```python
from build123d import *

# Parameters (mm, degrees)
BOSS_EXTRUDE1_START                 = 5
BOSS_EXTRUDE1_DEPTH                 = 5
BOSS_EXTRUDE2_START                 = 5
BOSS_EXTRUDE2_DEPTH                 = 5
BOSS_EXTRUDE3_START                 = 5
BOSS_EXTRUDE3_DEPTH                 = 5
F_1_5MM_DOWEL_HOLE1_D               = 1.5
F_1_5MM_DOWEL_HOLE1_DEPTH           = 3
F_1_5MM_DOWEL_HOLE1_TIP             = 0.450645464
F_1_5MM_DOWEL_HOLE1_ON_FACE_2_D     = 1.5
F_1_5MM_DOWEL_HOLE1_ON_FACE_2_DEPTH = 3
F_1_5MM_DOWEL_HOLE1_ON_FACE_2_TIP   = 0.450645464
F_1_5MM_DOWEL_HOLE1_ON_FACE_3_D     = 1.5
F_1_5MM_DOWEL_HOLE1_ON_FACE_3_DEPTH = 3
F_1_5MM_DOWEL_HOLE1_ON_FACE_3_TIP   = 0.450645464
F_1_5MM_DOWEL_HOLE1_ON_FACE_4_D     = 1.5
F_1_5MM_DOWEL_HOLE1_ON_FACE_4_DEPTH = 3
F_1_5MM_DOWEL_HOLE1_ON_FACE_4_TIP   = 0.450645464
F_1_5MM_DOWEL_HOLE1_ON_FACE_5_D     = 1.5
F_1_5MM_DOWEL_HOLE1_ON_FACE_5_DEPTH = 3
F_1_5MM_DOWEL_HOLE1_ON_FACE_5_TIP   = 0.450645464
F_1_5MM_DOWEL_HOLE1_ON_FACE_6_D     = 1.5
F_1_5MM_DOWEL_HOLE1_ON_FACE_6_DEPTH = 3
F_1_5MM_DOWEL_HOLE1_ON_FACE_6_TIP   = 0.450645464
CUT_EXTRUDE2_DEPTH                  = 4


with BuildPart() as part:
    # Sketch1 → Revolve1 (revolve)
    with BuildSketch(Plane.XY, mode=Mode.PRIVATE) as revolve1_sk:
        Polygon((54, 11), (55.5, 11), (55.5, -4), (48, -4), (48, -3), (54, -3), align=None)
    revolve(revolve1_sk.sketch.rotate(Axis((0, 0, 0), (0, 1, 0)), 90), axis=Axis((0, 0, 0), (0, 1, 0)))

    # Sketch3 → Boss-Extrude1 (add)
    with BuildSketch(Plane(origin=(0, -3, 0), x_dir=(1, 0, 0), z_dir=(0, 1, 0)).offset(BOSS_EXTRUDE1_START)):
        with BuildLine():
            Line((-16.686917696, -51.35705188), (-15.450849719, -47.552825815))
            ThreePointArc((-15.450849719, -47.552825815), (-25, -43.301270189), (-33.456530318, -37.157241274))
            Line((-33.456530318, -37.157241274), (-36.133052743, -40.129820576))
            ThreePointArc((-36.133052743, -40.129820576), (-27, -46.765371804), (-16.686917696, -51.35705188))
        make_face()
    extrude(amount=-BOSS_EXTRUDE1_DEPTH)

    # Sketch3_3 → Boss-Extrude2 (add)
    with BuildSketch(Plane(origin=(0, -3, 0), x_dir=(1, 0, 0), z_dir=(0, 1, 0)).offset(BOSS_EXTRUDE2_START)):
        with BuildLine():
            ThreePointArc((48.907380037, 10.395584541), (49.726094768, 5.226423163), (50, 0))
            ThreePointArc((50, 0), (49.726094768, -5.226423163), (48.907380037, -10.395584541))
            Line((48.907380037, -10.395584541), (52.81997044, -11.227231304))
            ThreePointArc((52.81997044, -11.227231304), (53.70418235, -5.644537016), (54, 0))
            ThreePointArc((54, 0), (53.70418235, 5.644537016), (52.81997044, 11.227231304))
            Line((52.81997044, 11.227231304), (48.907380037, 10.395584541))
        make_face()
    extrude(amount=-BOSS_EXTRUDE2_DEPTH)

    # Sketch3_4 → Boss-Extrude3 (add)
    with BuildSketch(Plane(origin=(0, -3, 0), x_dir=(1, 0, 0), z_dir=(0, 1, 0)).offset(BOSS_EXTRUDE3_START)):
        with BuildLine():
            Line((-36.133052743, 40.129820576), (-33.456530318, 37.157241274))
            ThreePointArc((-33.456530318, 37.157241274), (-25, 43.301270189), (-15.450849719, 47.552825815))
            Line((-15.450849719, 47.552825815), (-16.686917696, 51.35705188))
            ThreePointArc((-16.686917696, 51.35705188), (-27, 46.765371804), (-36.133052743, 40.129820576))
        make_face()
    extrude(amount=-BOSS_EXTRUDE3_DEPTH)

    # 1.5mm Dowel Hole1
    with Locations(Plane(origin=(-30.090751158, 0, -39.931775502), x_dir=(0.798635510047, 0, -0.601815023152), z_dir=(0.601815023152, 0, 0.798635510047))):
        with Locations((1e-09, 0)):
            Hole(F_1_5MM_DOWEL_HOLE1_D / 2, depth=F_1_5MM_DOWEL_HOLE1_DEPTH)
            with Locations((0, 0, -(F_1_5MM_DOWEL_HOLE1_DEPTH + F_1_5MM_DOWEL_HOLE1_TIP / 2))):  # 118° drill point
                Cone(0, F_1_5MM_DOWEL_HOLE1_D / 2, F_1_5MM_DOWEL_HOLE1_TIP, mode=Mode.SUBTRACT)

    # 1.5mm Dowel Hole1 on face 2
    with Locations(Plane(origin=(-19.536556424, 0, -46.025242673), x_dir=(0.92050492204, 0, -0.390730966908), z_dir=(0.390730966908, 0, 0.92050492204))):
        with Locations((-1e-09, 0)):
            Hole(F_1_5MM_DOWEL_HOLE1_ON_FACE_2_D / 2, depth=F_1_5MM_DOWEL_HOLE1_ON_FACE_2_DEPTH)
            with Locations((0, 0, -(F_1_5MM_DOWEL_HOLE1_ON_FACE_2_DEPTH + F_1_5MM_DOWEL_HOLE1_ON_FACE_2_TIP / 2))):  # 118° drill point
                Cone(0, F_1_5MM_DOWEL_HOLE1_ON_FACE_2_D / 2, F_1_5MM_DOWEL_HOLE1_ON_FACE_2_TIP, mode=Mode.SUBTRACT)

    # 1.5mm Dowel Hole1 on face 3
    with Locations(Plane(origin=(49.627307582, 0, -6.09346717), x_dir=(-0.121869023443, 0, -0.992546190928), z_dir=(-0.992546190928, 0, 0.121869023443))):
        with Locations((0, 0)):
            Hole(F_1_5MM_DOWEL_HOLE1_ON_FACE_3_D / 2, depth=F_1_5MM_DOWEL_HOLE1_ON_FACE_3_DEPTH)
            with Locations((0, 0, -(F_1_5MM_DOWEL_HOLE1_ON_FACE_3_DEPTH + F_1_5MM_DOWEL_HOLE1_ON_FACE_3_TIP / 2))):  # 118° drill point
                Cone(0, F_1_5MM_DOWEL_HOLE1_ON_FACE_3_D / 2, F_1_5MM_DOWEL_HOLE1_ON_FACE_3_TIP, mode=Mode.SUBTRACT)

    # 1.5mm Dowel Hole1 on face 4
    with Locations(Plane(origin=(49.627307582, 0, 6.09346717), x_dir=(0.121869023443, 0, -0.992546190928), z_dir=(-0.992546190928, 0, -0.121869023443))):
        with Locations((0, 0)):
            Hole(F_1_5MM_DOWEL_HOLE1_ON_FACE_4_D / 2, depth=F_1_5MM_DOWEL_HOLE1_ON_FACE_4_DEPTH)
            with Locations((0, 0, -(F_1_5MM_DOWEL_HOLE1_ON_FACE_4_DEPTH + F_1_5MM_DOWEL_HOLE1_ON_FACE_4_TIP / 2))):  # 118° drill point
                Cone(0, F_1_5MM_DOWEL_HOLE1_ON_FACE_4_D / 2, F_1_5MM_DOWEL_HOLE1_ON_FACE_4_TIP, mode=Mode.SUBTRACT)

    # 1.5mm Dowel Hole1 on face 5
    with Locations(Plane(origin=(-30.090751158, 0, 39.931775502), x_dir=(-0.798635698626, 0, -0.601814772899), z_dir=(0.601814772899, 0, -0.798635698626))):
        with Locations((-1e-09, 0)):
            Hole(F_1_5MM_DOWEL_HOLE1_ON_FACE_5_D / 2, depth=F_1_5MM_DOWEL_HOLE1_ON_FACE_5_DEPTH)
            with Locations((0, 0, -(F_1_5MM_DOWEL_HOLE1_ON_FACE_5_DEPTH + F_1_5MM_DOWEL_HOLE1_ON_FACE_5_TIP / 2))):  # 118° drill point
                Cone(0, F_1_5MM_DOWEL_HOLE1_ON_FACE_5_D / 2, F_1_5MM_DOWEL_HOLE1_ON_FACE_5_TIP, mode=Mode.SUBTRACT)

    # 1.5mm Dowel Hole1 on face 6
    with Locations(Plane(origin=(-19.536556424, 0, 46.025242673), x_dir=(-0.92050492204, 0, -0.390730966908), z_dir=(0.390730966908, 0, -0.92050492204))):
        with Locations((1e-09, 0)):
            Hole(F_1_5MM_DOWEL_HOLE1_ON_FACE_6_D / 2, depth=F_1_5MM_DOWEL_HOLE1_ON_FACE_6_DEPTH)
            with Locations((0, 0, -(F_1_5MM_DOWEL_HOLE1_ON_FACE_6_DEPTH + F_1_5MM_DOWEL_HOLE1_ON_FACE_6_TIP / 2))):  # 118° drill point
                Cone(0, F_1_5MM_DOWEL_HOLE1_ON_FACE_6_D / 2, F_1_5MM_DOWEL_HOLE1_ON_FACE_6_TIP, mode=Mode.SUBTRACT)

    # Sketch7 → Cut-Extrude2 (cut)
    with BuildSketch(Plane(origin=(0, 11, 0), x_dir=(1, 0, 0), z_dir=(0, 1, 0))):
        with BuildLine():
            Line((-17.150443188, -52.783636654), (-16.686917696, -51.35705188))
            ThreePointArc((-16.686917696, -51.35705188), (-27, -46.765371804), (-36.133052743, -40.129820576))
            Line((-36.133052743, -40.129820576), (-37.136748653, -41.244537814))
            ThreePointArc((-37.136748653, -41.244537814), (-27.75, -48.06440991), (-17.150443188, -52.783636654))
        make_face()
    extrude(amount=-CUT_EXTRUDE2_DEPTH, mode=Mode.SUBTRACT)


solid = part.part
```
Can you work these out from the model? Positions are in its coordinate system, mm. A direction names the side the tool comes from. Coordinates: 2 decimals unless noted, no trailing zeros. Loops run counter-clockwise (first coordinate to the right, second up) from the corner with the lowest first, then second, coordinate; pieces in that order, holes last. Notation, with made-up numbers: (18.25, 17.5) -> (55.25, 17.5) arc R17 cw to (55.25, 26.5) -> close; hole circle Ø6 at (20, 12). An arc over 180 degrees is marked (long way). Put each result on its own line as item: value. Start each with the question number.
Q1. Thinking about a two-plate mould opening in Z: for faces 1 (the face through (-16.671, 3.395, -52.937)), 2 (the face through (-41.4, -4, 24.9)), 3 (the face through (-24.873, -0.465, 43.374)), which applies, pulls with the +Z half, pulls with the -Z half, needs draft (parallel to the pull), parting line crosses it, or undercut?
Q2. I want a section at B-B (z = 18). Write out the boundary of the cut face in (x, y).
Q3. I'm going to push flat-ended pins straight in: P1, Ø3, axis at x = 25, y = 5, coming from the +Z side; P2, Ø3, axis at x = -32.5, y = 2.5, coming from the -Z side; P3, Ø3, axis at y = 5, z = 36, coming from the -X side; P4, Ø15.5, axis at x = -25.5, z = -47, coming from the +Y side. Where does each tip first touch, or does it pass through?
Q4. If I drill on line 1 (X direction, y = 3.25, z = 0); line 2 (X direction, y = -3.25, z = 0); line 3 (Y direction, x = 50.5, z = -16), over which ranges is the centre line in solid material (lowest first)? Write a range as [from, to].
Q5. For faces 4 (the face through (-30.43, 0.23, 41.57)), 5 (the face through (-16.06, -0.46, -49.43)), which set-ups out of +Z, -Z, +X, -X, +Y, -Y let a thin tool reach every point of the face, with its end or its side?
Q6. I want a section at A-A (x = 0). Write out the boundary of the cut face in (y, z).
Q7. I want a section at C-C (y = 4.5). Write out the boundary of the cut face in (x, z).
Taken from the geometry:
1. face 1: parting line crosses it
1. face 2: needs draft
1. face 3: undercut
2. outline: (-52.5, -4) -> (-44.5, -4) -> (-44.5, -3) -> (-50.91, -3) -> (-50.91, 11) -> (-52.5, 11) -> close; (44.5, -4) -> (52.5, -4) -> (52.5, 11) -> (50.91, 11) -> (50.91, -3) -> (44.5, -3) -> close
3. P1: stops at z = 50.28
3. P2: stops at z = -46.04
3. P3: stops at x = -43.47
3. P4: stops at y = 11
4. line 1: x = [-55.5, -54], [54, 55.5]
4. line 2: x = [-55.5, -48], [48, 55.5]
4. line 3: y = [-4, -3]
5. face 4: none
5. face 5: +Y
6. outline: (-4, -55.5) -> (11, -55.5) -> (11, -54) -> (-3, -54) -> (-3, -48) -> (-4, -48) -> close; (-4, 48) -> (-3, 48) -> (-3, 54) -> (11, 54) -> (11, 55.5) -> (-4, 55.5) -> close
7. outline: circle Ø111 at (0, 0); hole circle Ø108 at (0, 0)
